Input: part model. Units: mm. Frame: model coordinates. A direction names the side the tool comes from. Give positions to 0.01 mm unless a question says otherwise; leave off trailing zeros. Write each loop counter-clockwise with the first axis right and the second up, starting at its lowest first coordinate (ties: lowest second). Pieces come first, ordered by that corner, then holes.
```python
from build123d import *

# Parameters (mm, degrees)
BOSS_EXTRU_1_DEPTH                 = 8
ESQUISSE5_R                        = 14.567729557
BOSS_EXTRU_2_DEPTH                 = 8
CONG_1_R                           = 5
CONG_2_R                           = 5
R_P_TITION_CIRCULAIRE8_COUNT       = 5
CONG_1_OF_R_P_TITION_CIRCULAIRE8_R = 5
CONG_2_OF_R_P_TITION_CIRCULAIRE8_R = 5
ESQUISSE9_R                        = 10
BOSS_EXTRU_4_DEPTH                 = 5
ESQUISSE10_R                       = 5
BOSS_EXTRU_5_DEPTH                 = 5
ESQUISSE12_R                       = 5.2
ENL_V_MAT_EXTRU_3_DEPTH            = 6


with BuildPart() as part:
    # Esquisse4 → Boss.-Extru.1 (new body)
    with BuildSketch(Plane(origin=(0, 0, 0), x_dir=(1, 0, 0), z_dir=(0, 1, 0))):
        with BuildLine():
            Line((2.2, -20.318922986), (2.2, -10.266937226))
            ThreePointArc((2.2, -10.266937226), (10.190195312, -2.531781884), (6.749269902, 8.043466653))
            ThreePointArc((6.749269902, 8.043466653), (5.499269902, 7.46058208), (5.142300877, 6.128355545))
            ThreePointArc((5.142300877, 6.128355545), (0, -8), (-5.142300877, 6.128355545))
            ThreePointArc((-5.142300877, 6.128355545), (-5.499269902, 7.46058208), (-6.749269902, 8.043466653))
            ThreePointArc((-6.749269902, 8.043466653), (-10.190195312, -2.531781884), (-2.2, -10.266937226))
            Line((-2.2, -10.266937226), (-2.2, -20.318922986))
            ThreePointArc((-2.2, -20.318922986), (0, -20.179612502), (2.2, -20.318922986))
        make_face()
    boss_extru_1 = extrude(amount=BOSS_EXTRU_1_DEPTH)

    # Esquisse5 → Boss.-Extru.2 (add)
    with BuildSketch(Plane(origin=(0, 0, 0), x_dir=(1, 0, 0), z_dir=(0, 1, 0))):
        with Locations((0, -34.71957382)):
            Circle(ESQUISSE5_R)
    extrude(amount=BOSS_EXTRU_2_DEPTH)

    # Congé1
    cong_1_edges = [part.edges().sort_by_distance(p)[0] for p in [
        (2.2, 4, 10.266937226),
        (-2.2, 4, 10.266937226),
    ]]
    fillet(cong_1_edges, radius=CONG_1_R)

    # Congé2
    cong_2_edges = [part.edges().sort_by_distance(p)[0] for p in [
        (2.2, 4, 20.318922986),
        (-2.2, 4, 20.318922986),
    ]]
    fillet(cong_2_edges, radius=CONG_2_R)

    # Répétition circulaire8: Boss.-Extru.1 ×5 about axis
    r_p_tition_circulaire8_axis = Axis((0, 0, 34.71957382), (0, 1, 0))
    for i in range(1, R_P_TITION_CIRCULAIRE8_COUNT):
        add(boss_extru_1.rotate(r_p_tition_circulaire8_axis, i * 360 / R_P_TITION_CIRCULAIRE8_COUNT))

    # Congé1 of Répétition circulaire8
    cong_1_of_r_p_tition_circulaire8_edges = [part.edges().sort_by_distance(p)[0] for p in [
        (-22.576001986, 4, 25.070969219),
        (-23.935676761, 4, 29.255617891),
        (-16.152736557, 4, 53.209044827),
        (-12.593061782, 4, 55.795299938),
        (12.593061782, 4, 55.795299938),
        (16.152736557, 4, 53.209044827),
        (23.935676761, 4, 29.255617891),
        (22.576001986, 4, 25.070969219),
    ]]
    fillet(cong_1_of_r_p_tition_circulaire8_edges, radius=CONG_1_OF_R_P_TITION_CIRCULAIRE8_R)

    # Congé2 of Répétition circulaire8
    cong_2_of_r_p_tition_circulaire8_edges = [part.edges().sort_by_distance(p)[0] for p in [
        (-13.015995427, 4, 28.177203647),
        (-14.375670202, 4, 32.361852318),
        (-10.244327571, 4, 45.07681752),
        (-6.684652796, 4, 47.66307263),
        (6.684652796, 4, 47.66307263),
        (10.244327571, 4, 45.07681752),
        (14.375670202, 4, 32.361852318),
        (13.015995427, 4, 28.177203647),
    ]]
    fillet(cong_2_of_r_p_tition_circulaire8_edges, radius=CONG_2_OF_R_P_TITION_CIRCULAIRE8_R)

    # Esquisse9 → Boss.-Extru.4 (add)
    with BuildSketch(Plane.XZ):
        with Locations(Location((-0.001570364, 34.773487041, 0), (0, 0, 90))):
            Circle(ESQUISSE9_R)
    extrude(amount=BOSS_EXTRU_4_DEPTH)

    # Esquisse10 → Boss.-Extru.5 (add)
    with BuildSketch(Plane.XZ.offset(5)):
        with Locations(Location((0, 35.07133439, 0), (0, 0, 270))):
            Circle(ESQUISSE10_R)
    extrude(amount=BOSS_EXTRU_5_DEPTH)

    # Esquisse12 → Enlèv. mat.-Extru.3 (cut)
    with BuildSketch(Plane(origin=(0, 8, 0), x_dir=(1, 0, 0), z_dir=(0, 1, 0))):
        with Locations(Location((-0.060638465, -34.698547828, 0), (0, 0, 270))):
            Circle(ESQUISSE12_R)
    extrude(amount=-ENL_V_MAT_EXTRU_3_DEPTH, mode=Mode.SUBTRACT)


solid = part.part
```
Q1. Section B-B, the plane x = -35.5. Return the cut outline in (y, z), then the cut area to 3 significant figures.
Q2. Section D-D, the plane y = -8. Return the cut outline in (x, z).
Q3. Access query for faces 1 (the cylindrical face through (-13.87, 3.94, 39.17)), 2 (the cylindrical face through (10.423, 3.944, 1.27)), 3 (the cylindrical face through (21.5, 4.06, 24.68)), 4 (the cylindrical face through (-3.09, 4.06, 19.37)). Directions: +Z, -Z, +X, -X, +Y, -Y. A direction counts if a zero-diameter tool reaches every point of the face in a straight line with its end or side. Return the directions, or none.
Q4. Section C-C, the plane z = 38. Return the cut outline in (x, y).
Q5. Mould query, pull axis X, two halves, no side actions, for faces 5 (the cylindrical face through (13.72, 4.06, 27.06)), 6 (the cylindrical face through (13.84, 3.94, 39.27)), 7 (the flat face through (6, 0, 26)). Classes: +X half, -X half, draft (parallel to the pull), parting line (faces both ways), or undercut.
Q6. Pin query (flat end, axial travel): pin 1 (3 mm diameter, centred on y = 5, z = 15.5, fed in from -X); pin 2 (1.5 mm diameter, centred on y = 3, z = 35.5, fed in from +X); pin 3 (18.5 mm diameter, centred on x = 33.02, z = 23.99, fed in from -Y). Return the tip coordinate at first contact, or that it passes through.
Q7. Material intervals for line 1 along Z through (x, y) = (0, 4); line 2 along X through (y, z) = (6.25, 0); line 3 along X through (y, z) = (7, 24.5), sorted ascending.
Q8. Section A-A, the plane z = 0. Return the cut outline in (x, y), then the cut area to 3 significant figures.
Solutions:
1. outline: (0, 13.79) - (8, 13.79) - (8, 16.38) - (0, 16.38) - close; (0, 31.6) - (8, 31.6) - (8, 34.19) - (0, 34.19) - close
1. area: 41.6 mm2
2. outline: circle Ø10 at (0, 35.07)
3. face 1: -X, +Y, -Y
3. face 2: +X, +Y, -Y
3. face 3: -Z, +Y, -Y
3. face 4: +Y, -Y
4. outline: (-14.19, 0) - (-9.47, 0) - (-9.47, -5) - (-4.05, -5) - (-4.05, -10) - (4.05, -10) - (4.05, -5) - (9.46, -5) - (9.46, 0) - (14.19, 0) - (14.19, 8) - (3.96, 8) - (3.96, 2) - (-4.08, 2) - (-4.08, 8) - (-14.19, 8) - close
5. face 5: undercut
5. face 6: +X half
5. face 7: draft
6. pin 1: stops at x = -38.66
6. pin 2: stops at x = 14.67
6. pin 3: stops at y = 0
7. line 1: z = 8 to 29.5, 39.9 to 49.29
7. line 2: x = -10.5 to -8, 8 to 10.5
7. line 3: x = -25.04 to -21.65, -10.38 to 10.38, 21.65 to 25.04
8. outline: (-10.5, 0) - (-8, 0) - (-8, 8) - (-10.5, 8) - close; (8, 0) - (10.5, 0) - (10.5, 8) - (8, 8) - close
8. area: 40.0 mm2
